Answer from the drawing. Dimensions are ordinates in mm from the lowest x, y and z of the part. Coordinates: 2 decimals unless noted, no trailing zeros. Order: outer loops, then holes, each group sorted by start corner. A loop starts at its lowest first (then second) coordinate and runs counter-clockwise, first axis right, second up. Notation, with made-up numbers: (77.25, -29) -> (94.25, -29) arc R17 ccw to (94.25, 0) -> close; hole circle Ø7 at (51, -28.75). An arc over 180 degrees is marked (long way). Answer in a Markdown table with one row per item.
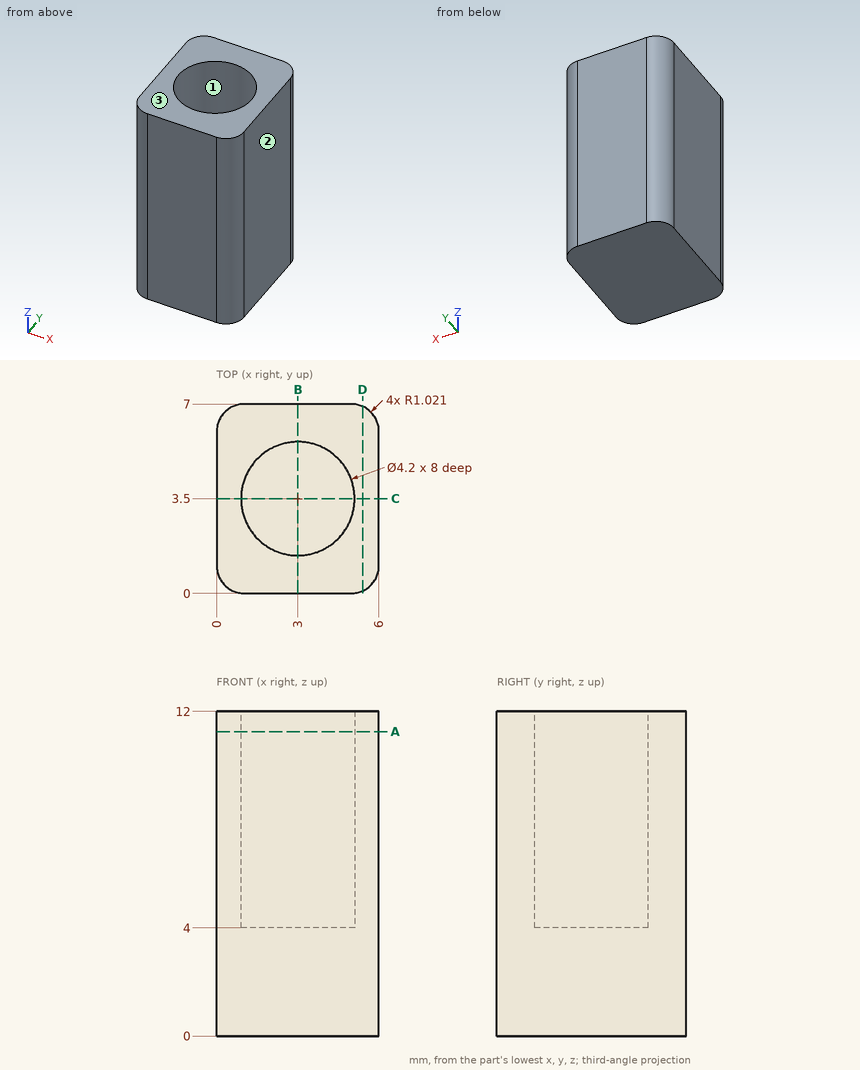
Q1. For a pull along X with two mould halves and no side action, classify the marked faces 1, 2 and 3 as pulls with the +X half, pulls with the -X half, needs draft (parallel to the pull), parting line crosses it, or undercut.
Outcome:
| item | result |
|---|---|
| face 1 | undercut |
| face 2 | pulls with the +X half |
| face 3 | needs draft |
Q2. Given pin 1 (2.5 mm diameter, centred on x = 3, y = 3.5, fed in from +Z), flat-ended and moving along its own axis, determine where the tip first touches the part or whether it passes through.
Outcome:
| item | result |
|---|---|
| pin 1 | z = 4 |
Q3. The part is cut by section B-B (x = 3). Write down the section's boundary in (y, z).
Outcome:
| item | result |
|---|---|
| outline | (0, 0) -> (7, 0) -> (7, 12) -> (5.6, 12) -> (5.6, 4) -> (1.4, 4) -> (1.4, 12) -> (0, 12) -> close |
Q4. The part is cut by section D-D (x = 5.4). Write down the section's boundary in (y, z), then the cut area to 3 significant figures.
Outcome:
| item | result |
|---|---|
| outline | (0.09, 0) -> (6.91, 0) -> (6.91, 12) -> (0.09, 12) -> close |
| area | 81.8 mm² |
Q5. Consider line 1 (Y direction, x = 3, z = 9); line 2 (Z direction, x = 2.05, y = 3); line 3 (X direction, y = 4.5, z = 4.75). Determine where each line is inside the solid, lowest interval first.
Outcome:
| item | result |
|---|---|
| line 1 | 0 to 1.4, 5.6 to 7 |
| line 2 | 0 to 4 |
| line 3 | 0 to 1.15, 4.85 to 6 |
Q6. The part is cut by section A-A (z = 11.25). Write down the section's boundary in (x, y).
Outcome:
| item | result |
|---|---|
| outline | (0, 1.02) arc R1.02 ccw to (1.02, 0) -> (4.98, 0) arc R1.02 ccw to (6, 1.02) -> (6, 5.98) arc R1.02 ccw to (4.98, 7) -> (1.02, 7) arc R1.02 ccw to (0, 5.98) -> close; hole circle Ø4.2 at (3, 3.5) |
Q7. The part is cut by section C-C (y = 3.5). Write down the section's boundary in (x, z).
Outcome:
| item | result |
|---|---|
| outline | (0, 0) -> (6, 0) -> (6, 12) -> (5.1, 12) -> (5.1, 4) -> (0.9, 4) -> (0.9, 12) -> (0, 12) -> close |
